The model under review builds one solid part; all positions refer to its coordinate system, in mm. Face numbers are marked on the shaded views. A direction names the side the tool comes from. Round coordinates to 2 decimals unless told otherwise and drop trailing zeros. Write each loop counter-clockwise with the first axis right and the second up, starting at its lowest first coordinate (ties: lowest second). Pieces come first, ordered by that corner, then holes. Notation, with made-up numbers: (1.5, 82) -> (25.5, 82) arc R29 ccw to (25.5, 106) -> close; hole circle Ø3 at (-4.75, -2). An arc over 180 degrees is marked (long way). Return JSON: item names as keys, results as strings. Group by question number.
1. For line 1 along X through (y, z) = (-2.5, 21.5); line 2 along X through (y, z) = (-25.5, 29.5); line 3 along X through (y, z) = (-1.5, 1), list the stretches that pass through material, from the lowest coordinate up. Write a range as from..to.
2. Take a section at A-A, the plane y = 0. Write out the cut boundary in (x, z).
3. Mouldability with a two-part tool opening along Y and no side actions: class the marked faces 5, 6, 7 and 8 as pulls with the +Y half, pulls with the -Y half, needs draft (parallel to the pull), parting line crosses it, or undercut.
4. Tool access review of the marked faces 1, 2, 3 and 4: name each direction out of +Z, -Z, +X, -X, +Y, -Y from which nothing blocks a thin tool from reaching the whole face with its end or side.
5. Take a section at D-D, the plane y = -49. Write out the cut boundary in (x, z) (3 decimals), then the cut area to 3 significant figures.
6. Clearance check with flat-ended pins moving along their axes: P1, Ø1.8, axis at x = 26.5, z = 22.5, coming from the -Y side; P2, Ø5, axis at x = 12.5, y = 1.5, coming from the -Z side; P3, Ø1.5, axis at x = 6.5, z = -2.5, coming from the -Y side; P4, Ø8, axis at y = -15, z = -8, coming from the +X side. State where each tip first meets the part, or that it passes through.
7. Take a section at B-B, the plane x = -33.8. Write out the cut boundary in (y, z).
8. Take a section at C-C, the plane x = 0. Write out the cut boundary in (y, z), then the cut area to 3 significant figures.
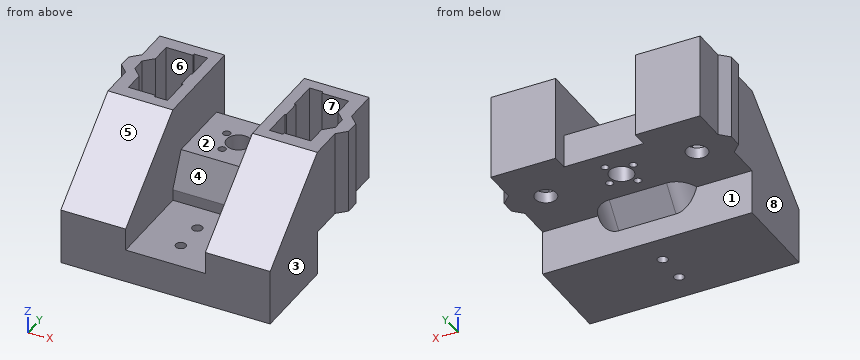
from build123d import *

# Parameters (mm, degrees)
CROQUIS1_R               = 6
SALIENTE_EXTRUIR1_DEPTH  = 38
CROQUIS4_R               = 4.75
SALIENTE_EXTRUIR3_DEPTH  = 5
CROQUIS7_R               = 6
CROQUIS7_R_2             = 5.35
SALIENTE_EXTRUIR4_DEPTH  = 38
CROQUIS8_R               = 1.65
CORTAR_EXTRUIR3_DEPTH    = 38
CROQUIS9_W               = 35.6
CROQUIS9_H               = 23
CORTAR_EXTRUIR4_DEPTH    = 74.441405215
CROQUIS10_W              = 93.6
CROQUIS10_H              = 5
SALIENTE_EXTRUIR5_DEPTH  = 40
CROQUIS11_R              = 2.25
CORTAR_EXTRUIR5_DEPTH    = 87.681255182
CROQUIS14_R              = 2.25
SALIENTE_EXTRUIR6_DEPTH  = 20
SALIENTE_EXTRUIR7_START  = -29
SALIENTE_EXTRUIR7_DEPTH  = 29
SALIENTE_EXTRUIR8_START  = -29
SALIENTE_EXTRUIR8_DEPTH  = 29
CROQUIS17_W              = 35.6
CROQUIS17_H              = 10
CORTAR_EXTRUIR6_DEPTH    = 40
CROQUIS23_W              = 45.6
CROQUIS23_H              = 10
SALIENTE_EXTRUIR11_DEPTH = 8
CORTAR_EXTRUIR7_DEPTH    = 104.464776615
REDONDEO4_R              = 10
SALIENTE_EXTRUIR12_DEPTH = 35.6


with BuildPart() as part:
    # Croquis1 → Saliente-Extruir1 (new body)
    with BuildSketch(Plane.XY):
        Polygon((-50.8, -3), (-50.8, 3), (-46.8, 7), (-46.8, 22), (-17.8, 22), (-17.8, 15), (17.8, 15), (17.8, 22), (46.8, 22), (46.8, 7), (50.8, 3), (50.8, -3), (46.8, -7), (46.8, -22), (17.8, -22), (17.8, -15), (-17.8, -15), (-17.8, -22), (-46.8, -22), (-46.8, -7), align=None)
        Circle(CROQUIS1_R, mode=Mode.SUBTRACT)
        Polygon((-22.8, 4), (-23.45, 4), (-23.45, -4), (-22.8, -4), (-22.8, -17), (-28.8, -17), (-28.8, -16), (-40.8, -16), (-40.8, -7), (-44.8, -3), (-44.8, 3), (-40.8, 7), (-40.8, 16), (-28.8, 16), (-28.8, 17), (-22.8, 17), align=None, mode=Mode.SUBTRACT)
        Polygon((23.45, -4), (23.45, 4), (22.8, 4), (22.8, 17), (28.8, 17), (28.8, 16), (40.8, 16), (40.8, 7), (44.8, 3), (44.8, -3), (40.8, -7), (40.8, -16), (28.8, -16), (28.8, -17), (22.8, -17), (22.8, -4), align=None, mode=Mode.SUBTRACT)
    extrude(amount=SALIENTE_EXTRUIR1_DEPTH)

    # Croquis4 → Saliente-Extruir3 (add)
    # profile 1 of 2: a face of its own
    with BuildSketch(Plane(origin=(0, 0, 0), x_dir=(-1, 0, 0), z_dir=(0, 0, -1))):
        Polygon((-40.8, 16), (-28.8, 16), (-28.8, 17), (-22.8, 17), (-22.8, 4), (-23.45, 4), (-23.45, -4), (-22.8, -4), (-22.8, -17), (-28.8, -17), (-28.8, -16), (-40.8, -16), (-40.8, -7), (-44.8, -3), (-44.8, 3), (-40.8, 7), align=None)
        with Locations((-33.8, 0)):
            Circle(CROQUIS4_R, mode=Mode.SUBTRACT)
    # profile 2 of 2: a face of its own
    with BuildSketch(Plane(origin=(0, 0, 0), x_dir=(-1, 0, 0), z_dir=(0, 0, -1))):
        Polygon((40.8, 7), (40.8, 16), (28.8, 16), (28.8, 17), (22.8, 17), (22.8, 4), (23.45, 4), (23.45, -4), (22.8, -4), (22.8, -17), (28.8, -17), (28.8, -16), (40.8, -16), (40.8, -7), (44.8, -3), (44.8, 3), align=None)
        with Locations(Location((33.8, 0, 0), (0, 0, 180))):
            Circle(CROQUIS4_R, mode=Mode.SUBTRACT)
    extrude(amount=-SALIENTE_EXTRUIR3_DEPTH)

    # Croquis7 → Saliente-Extruir4 (add)
    with BuildSketch(Plane(origin=(0, 0, 0), x_dir=(-1, 0, 0), z_dir=(0, 0, -1))):
        Circle(CROQUIS7_R)
        Circle(CROQUIS7_R_2, mode=Mode.SUBTRACT)
    extrude(amount=-SALIENTE_EXTRUIR4_DEPTH)

    # Croquis8 → Cortar-Extruir3 (cut)
    with BuildSketch(Plane(origin=(0, 0, 0), x_dir=(-1, 0, 0), z_dir=(0, 0, -1))):
        with Locations((-7.15441776, -3.579707868)):
            Circle(CROQUIS8_R)
        with Locations((3.579707868, -7.15441776)):
            Circle(CROQUIS8_R)
        with Locations((7.15441776, 3.579707868)):
            Circle(CROQUIS8_R)
        with Locations((-3.579707868, 7.15441776)):
            Circle(CROQUIS8_R)
    extrude(amount=-CORTAR_EXTRUIR3_DEPTH, mode=Mode.SUBTRACT)

    # Croquis9 → Cortar-Extruir4 (cut, through all)
    with BuildSketch(Plane.XZ.offset(15)):
        with Locations((0, 26.5)):
            Rectangle(CROQUIS9_W, CROQUIS9_H)
    extrude(amount=-CORTAR_EXTRUIR4_DEPTH, mode=Mode.SUBTRACT)

    # Croquis10 → Saliente-Extruir5 (add)
    with BuildSketch(Plane.XZ.offset(22)):
        with Locations((0, 2.5)):
            Rectangle(CROQUIS10_W, CROQUIS10_H)
    extrude(amount=SALIENTE_EXTRUIR5_DEPTH)

    # Croquis11 → Cortar-Extruir5 (cut, through all)
    with BuildSketch(Plane.XY.offset(5)):
        with Locations((0, -35)):
            Circle(CROQUIS11_R)
        with Locations((0, -49)):
            Circle(CROQUIS11_R)
    extrude(amount=-CORTAR_EXTRUIR5_DEPTH, mode=Mode.SUBTRACT)

    # Croquis14 → Saliente-Extruir6 (add)
    with BuildSketch(Plane(origin=(0, 0, 0), x_dir=(-1, 0, 0), z_dir=(0, 0, -1))):
        Polygon((17.8, -22), (46.8, -22), (46.8, -62), (-46.8, -62), (-46.8, -22), align=None)
        with Locations(Location((0, -35, 0), (0, 0, 180))):
            Circle(CROQUIS14_R, mode=Mode.SUBTRACT)
        with Locations(Location((0, -49, 0), (0, 0, 180))):
            Circle(CROQUIS14_R, mode=Mode.SUBTRACT)
    extrude(amount=SALIENTE_EXTRUIR6_DEPTH)

    # Croquis15 → Saliente-Extruir7 (add)
    with BuildSketch(Plane.ZY.offset(46.8).offset(SALIENTE_EXTRUIR7_START)):
        Polygon((38, -22), (5, -62), (5, -22), align=None)
    extrude(amount=SALIENTE_EXTRUIR7_DEPTH)

    # Croquis16 → Saliente-Extruir8 (add)
    with BuildSketch(Plane(origin=(46.8, 0, 0), x_dir=(0, 0, -1), z_dir=(1, 0, 0)).offset(SALIENTE_EXTRUIR8_START)):
        Polygon((-38, -22), (-5, -62), (-5, -22), align=None)
    extrude(amount=SALIENTE_EXTRUIR8_DEPTH)

    # Croquis17 → Cortar-Extruir6 (cut)
    with BuildSketch(Plane.XZ.offset(62)):
        Rectangle(CROQUIS17_W, CROQUIS17_H)
    extrude(amount=-CORTAR_EXTRUIR6_DEPTH, mode=Mode.SUBTRACT)

    # Croquis23 → Saliente-Extruir11 (add)
    with BuildSketch(Plane(origin=(0, -22, 0), x_dir=(1, 0, 0), z_dir=(0, 1, 0))):
        with Locations((0, 5)):
            Rectangle(CROQUIS23_W, CROQUIS23_H)
    extrude(amount=SALIENTE_EXTRUIR11_DEPTH)

    # Croquis24 → Cortar-Extruir7 (cut, through all)
    with BuildSketch(Plane.ZY.offset(22.8)):
        Polygon((-10, -22), (0, -14), (-10, -14), align=None)
    extrude(amount=-CORTAR_EXTRUIR7_DEPTH, mode=Mode.SUBTRACT)

    # Redondeo4
    # the kernel refuses this fillet: 10 mm, written as the material it takes off along each edge
    with BuildSketch(Plane(origin=(-22.8, -37.617376189, -29.521720236), x_dir=(1, 0, 0), z_dir=(0, 0.6246950475544245, 0.7808688094430302))) as redondeo4_piece_1_section:
        with BuildLine():
            CenterArc((REDONDEO4_R, -REDONDEO4_R), REDONDEO4_R, 90, 90)
            Line((0, -REDONDEO4_R), (0, 0))
            Line((0, 0), (REDONDEO4_R, 0))
        make_face()
    redondeo4_piece_1 = extrude(amount=62.806248475, mode=Mode.PRIVATE)
    redondeo4_piece_1 = split(redondeo4_piece_1, bisect_by=Plane(origin=(-20.122466275, -22, -4.721973229), z_dir=(0, 1, 0)), keep=Keep.TOP, mode=Mode.PRIVATE)
    redondeo4_piece_1 = split(redondeo4_piece_1, bisect_by=Plane(origin=(-20.122466275, -19.662128578, 0), z_dir=(0, 0, -1)), keep=Keep.TOP, mode=Mode.PRIVATE)
    add(redondeo4_piece_1, mode=Mode.SUBTRACT)
    with BuildSketch(Plane(origin=(22.8, -37.617376189, -29.521720236), x_dir=(0, -0.7808688094430302, 0.6246950475544245), z_dir=(0, 0.6246950475544245, 0.7808688094430302))) as redondeo4_piece_2_section:
        with BuildLine():
            CenterArc((REDONDEO4_R, -REDONDEO4_R), REDONDEO4_R, 90, 90)
            Line((0, -REDONDEO4_R), (0, 0))
            Line((0, 0), (REDONDEO4_R, 0))
        make_face()
    redondeo4_piece_2 = extrude(amount=62.806248475, mode=Mode.PRIVATE)
    redondeo4_piece_2 = split(redondeo4_piece_2, bisect_by=Plane(origin=(20.122466276, -22, -4.72197323), z_dir=(0, 1, 0)), keep=Keep.TOP, mode=Mode.PRIVATE)
    redondeo4_piece_2 = split(redondeo4_piece_2, bisect_by=Plane(origin=(20.122466276, -19.662128579, 0), z_dir=(0, 0, -1)), keep=Keep.TOP, mode=Mode.PRIVATE)
    add(redondeo4_piece_2, mode=Mode.SUBTRACT)

    # Croquis25 → Saliente-Extruir12 (add)
    with BuildSketch(Plane.ZY.offset(-17.8)):
        Polygon((0, -22), (15, -15), (0, -15), align=None)
    extrude(amount=SALIENTE_EXTRUIR12_DEPTH)


solid = part.part
Output:
{
 "1": {"line 1": "x = -50.8..-44.8, -23.45..-17.8, 17.8..23.45, 44.8..50.8", "line 2": "x = -46.8..-17.8, 17.8..46.8", "line 3": "x = -50.8..-38.31, -29.29..-5.14, 5.14..29.29, 38.31..50.8"},
 "2": {"outline": "(-50.8, 0) -> (-38.55, 0) -> (-38.55, 5) -> (-44.8, 5) -> (-44.8, 38) -> (-50.8, 38) -> close; (-29.05, 0) -> (-5.35, 0) -> (-5.35, 15) -> (-17.8, 15) -> (-17.8, 38) -> (-23.45, 38) -> (-23.45, 5) -> (-29.05, 5) -> close; (5.35, 0) -> (29.05, 0) -> (29.05, 5) -> (23.45, 5) -> (23.45, 38) -> (17.8, 38) -> (17.8, 15) -> (5.35, 15) -> close; (38.55, 0) -> (50.8, 0) -> (50.8, 38) -> (44.8, 38) -> (44.8, 5) -> (38.55, 5) -> close"},
 "3": {"face 5": "pulls with the -Y half", "face 6": "undercut", "face 7": "undercut", "face 8": "needs draft"},
 "4": {"face 1": "-Z, +Y", "face 2": "+Z, +Y, -Y", "face 3": "+Z, -Z, +X, -Y", "face 4": "+Z, -Y"},
 "5": {"outline": "(-46.8, -20) -> (-2.25, -20) -> (-2.25, -5) -> (-17.8, -5) -> (-17.8, 15.725) -> (-46.8, 15.725) -> close; (2.25, -20) -> (46.8, -20) -> (46.8, 15.725) -> (17.8, 15.725) -> (17.8, -5) -> (2.25, -5) -> close", "area": "2,540 mm^2"},
 "6": {"P1": "stops at y = -41.88", "P2": "stops at z = 0", "P3": "stops at y = -22", "P4": "passes through"},
 "7": {"outline": "(-62, -20) -> (-22, -20) -> (-22, 0) -> (-4.75, 0) -> (-4.75, 5) -> (-16, 5) -> (-16, 38) -> (-22, 38) -> (-62, 5) -> close; (4.75, 0) -> (22, 0) -> (22, 38) -> (16, 38) -> (16, 5) -> (4.75, 5) -> close"},
 "8": {"outline": "(-62, -20) -> (-51.25, -20) -> (-51.25, -5) -> (-62, -5) -> close; (-46.75, -20) -> (-37.25, -20) -> (-37.25, -5) -> (-46.75, -5) -> close; (-32.75, -20) -> (-22, -20) -> (-22, -10) -> (-14, 0) -> (-5.35, 0) -> (-5.35, 15) -> (-15, 15) -> (-22, 0) -> (-22, -5) -> (-32.75, -5) -> close; (5.35, 0) -> (15, 0) -> (15, 15) -> (5.35, 15) -> close", "area": "847 mm^2"}
}
